from build123d import *

# Parameters (mm, degrees)
F1_DEPTH = 0.5
F3_DEPTH = 0.501


with BuildPart() as f1:
    # F0 (on Top) → F1 (new body)
    with BuildSketch(Plane.XY):
        Polygon((6.25, -10.825318), (12.5, 0), (6.25, 10.825318), (-6.25, 10.825318), (-12.5, 0), (-6.25, -10.825318), align=None)
    extrude(amount=F1_DEPTH)

    # F2 (on face) → F3 (cut, through all)
    with BuildSketch(Plane.XY.offset(0.5)):
        with BuildLine():
            ThreePointArc((4.4, -10.825318), (4.224264, -10.401053), (3.8, -10.225318))
            Line((3.8, -10.225318), (3.3, -10.225318))
            ThreePointArc((3.3, -10.225318), (2.875736, -10.401053), (2.7, -10.825318))
            Line((2.7, -10.825318), (4.4, -10.825318))
        make_face()
        with BuildLine():
            ThreePointArc((0.85, -10.825318), (0.674264, -10.401053), (0.25, -10.225318))
            Line((0.25, -10.225318), (-0.25, -10.225318))
            ThreePointArc((-0.25, -10.225318), (-0.674264, -10.401053), (-0.85, -10.825318))
            Line((-0.85, -10.825318), (0.85, -10.825318))
        make_face()
        with BuildLine():
            ThreePointArc((-2.7, -10.825318), (-2.875736, -10.401053), (-3.3, -10.225318))
            Line((-3.3, -10.225318), (-3.8, -10.225318))
            ThreePointArc((-3.8, -10.225318), (-4.224264, -10.401053), (-4.4, -10.825318))
            Line((-4.4, -10.825318), (-2.7, -10.825318))
        make_face()
    extrude(amount=-F3_DEPTH, mode=Mode.SUBTRACT)


solid = f1.part
Here's how the part is built. I have some questions about the finished solid (model axes, mm). Give positions to 0.01 mm unless a question says otherwise; leave off trailing zeros. Loops run counter-clockwise (first coordinate to the right, second up) from the corner with the lowest first, then second, coordinate; pieces in that order, holes last. Notation, with made-up numbers: (38.5, -27) -> (60.5, -27) arc R21 ccw to (60.5, 9) -> close; hole circle Ø5 at (59, 79). An arc over 180 degrees is marked (long way). Answer as a JSON object with one key per item and string values. Group by question number.
Item 1: Imagine slicing it at A-A on z = 0.3. Write out the boundary of the cut face in (x, y), then the cut area to 3 significant figures.
Item 2: Imagine slicing it at B-B on y = -3.25. Write out the boundary of the cut face in (x, z), then the cut area to 3 significant figures.
Item 3: I need wall thicknesses on L1, parallel to Y at x = 7.75, z = 0.25; L2, parallel to X at y = 2.25, z = 0.3; L3, parallel to Y at x = -4, z = 0.2. Which ranges of each line are inside material? Lowest first, please.
Item 4: Imagine slicing it at C-C on x = -9.25. Write out the boundary of the cut face in (y, z).
Answer list:
{
 "1": {"outline": "(-12.5, 0) -> (-6.25, -10.83) -> (-4.4, -10.83) arc R0.6 cw to (-3.8, -10.23) -> (-3.3, -10.23) arc R0.6 cw to (-2.7, -10.83) -> (-0.85, -10.83) arc R0.6 cw to (-0.25, -10.23) -> (0.25, -10.23) arc R0.6 cw to (0.85, -10.83) -> (2.7, -10.83) arc R0.6 cw to (3.3, -10.23) -> (3.8, -10.23) arc R0.6 cw to (4.4, -10.83) -> (6.25, -10.83) -> (12.5, 0) -> (6.25, 10.83) -> (-6.25, 10.83) -> close", "area": "403 mm2"},
 "2": {"outline": "(-10.62, 0) -> (10.62, 0) -> (10.62, 0.5) -> (-10.62, 0.5) -> close", "area": "10.6 mm2"},
 "3": {"L1": "y = -8.23 to 8.23", "L2": "x = -11.2 to 11.2", "L3": "y = -10.26 to 10.83"},
 "4": {"outline": "(-5.63, 0) -> (5.63, 0) -> (5.63, 0.5) -> (-5.63, 0.5) -> close"}
}
